Autodesk Fusion 360 part; units mm, degrees
sketch "Sketch1" plane through (0, 0, 0) normal (0, 0, 1) x (1, 0, 0)
  line L0 (19.75, 4.5) -> (-19.75, 4.5)
  line L1 (-19.75, 4.5) -> (-19.75, -4.5)
  line L2 (-19.75, -4.5) -> (19.75, -4.5)
  line L3 (19.75, -4.5) -> (19.75, 4.5)
  line L4 (19.75, 4.5) -> (-19.75, -4.5) construction
  line L5 (-19.75, 4.5) -> (19.75, -4.5) construction
  dimension "d1" = 39.5
  dimension "d2" = 9
extrude "Extrude1" add sketch "Sketch1" along normal blind 2
fillet "Fillet1" radius 2.5 4 edges at (-19.75, -4.5, 1) (-19.75, 4.5, 1) (19.75, 4.5, 1) (19.75, -4.5, 1)
sketch "Sketch2" plane through (0, 0, 2) normal (0, 0, 1) x (-1, 0, 0)
  arc A0 (-17.25, 4.5) -> (-19.75, 2) centre (-17.25, 2) ccw
  line L0 (-17.25, -4.5) -> (17.25, -4.5)
  arc A1 (17.25, -4.5) -> (19.75, -2) centre (17.25, -2) ccw
  line L1 (17.25, 4.5) -> (-17.25, 4.5)
  line L2 (-19.75, 2) -> (-19.75, -2)
  arc A2 (-19.75, -2) -> (-17.25, -4.5) centre (-17.25, -2) ccw
  line L3 (19.75, -2) -> (19.75, 2)
  arc A3 (19.75, 2) -> (17.25, 4.5) centre (17.25, 2) ccw
  line L4 (19.75, 0) -> (-19.75, 0) construction
  line L5 (19.75, 0) -> (15.25, 0)
  line L6 (-19.75, 0) -> (-15.25, 0)
  circle A4 centre (15.25, 0) radius 2.7
  circle A5 centre (-15.25, 0) radius 2.7
  dimension "d11" = 4.5
  dimension "d12" = 4.5
  dimension "d13" = 5.4
  dimension "d14" = 5.4
extrude "Extrude2" cut sketch "Sketch2" against normal blind 3 contours A5 | A4
CAD build for the part. Positions are in the model's coordinates, mm. Round coordinates to 2 decimals unless told otherwise and drop trailing zeros. Loops run counter-clockwise (first coordinate to the right, second up) from the corner with the lowest first, then second, coordinate; pieces in that order, holes last. Notation, with made-up numbers: M -18,2 L 0,2 A27 ccw 0,23 Z; hole C -3.75,78 d6. An arc over 180 degrees is marked long. Return JSON: item names as keys, results as strings. Group by question number.
(1) Saw through at C-C, the plane y = 0. List the corners of the cut face in (x, z).
(2) Mould opens along Y. For faces 1 (the flat face through (-19.75, 0, 1)), 2 (the cylindrical face through (-17.825, -0.811, 1.014)), 3 (the cylindrical face through (19.037, 3.748, 1.014)), 4 (the cylindrical face through (-19.037, -3.748, 1.014)) say: +Y half, -Y half, draft (parallel to the pull), parting line (faces both ways), or undercut.
(3) Saw through at A-A, the plane x = -15.25. List the corners of the cut face in (y, z).
(4) Wall check: probe 1 along X at (y, z) = (0, 1.4); probe 2 along X at (y, z) = (2.25, 1.7); probe 3 along Y at (x, z) = (-15.25, 0.45). Give the ranges that are in metal, low to high. Write a range as [from, to].
(5) Saw through at B-B, the plane z = 0.5. List the corners of the cut face in (x, y), and give its area (3 significant figures).
Answer list:
{
 "1": {"outline": "M -19.75,0 L -17.95,0 L -17.95,2 L -19.75,2 Z; M -12.55,0 L 12.55,0 L 12.55,2 L -12.55,2 Z; M 17.95,0 L 19.75,0 L 19.75,2 L 17.95,2 Z"},
 "2": {"face 1": "draft", "face 2": "undercut", "face 3": "+Y half", "face 4": "-Y half"},
 "3": {"outline": "M -4.5,0 L -2.7,0 L -2.7,2 L -4.5,2 Z; M 2.7,0 L 4.5,0 L 4.5,2 L 2.7,2 Z"},
 "4": {"probe 1": "[-19.75, -17.95], [-12.55, 12.55], [17.95, 19.75]", "probe 2": "[-19.74, -16.74], [-13.76, 13.76], [16.74, 19.74]", "probe 3": "[-4.5, -2.7], [2.7, 4.5]"},
 "5": {"outline": "M -19.75,-2 A2.5 ccw -17.25,-4.5 L 17.25,-4.5 A2.5 ccw 19.75,-2 L 19.75,2 A2.5 ccw 17.25,4.5 L -17.25,4.5 A2.5 ccw -19.75,2 Z; hole C -15.25,0 d5.4; hole C 15.25,0 d5.4", "area": "304 mm2"}
}
